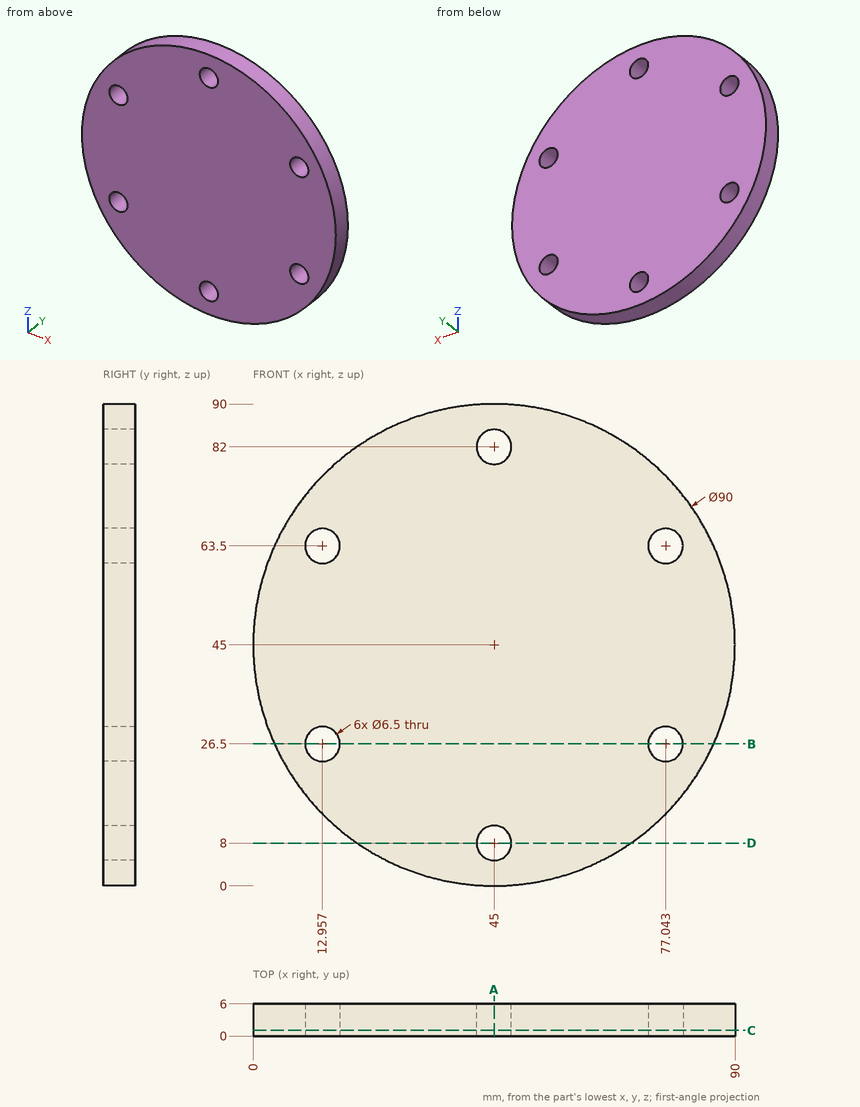
Here's the drawing with two shaded views (mm, measured from the low corner). I have some questions. Give positions to 0.01 mm unless a question says otherwise; leave off trailing zeros. Loops run counter-clockwise (first coordinate to the right, second up) from the corner with the lowest first, then second, coordinate; pieces in that order, holes last. Notation, with made-up numbers: (-5.75, 11.5) -> (13.25, 11.5) arc R15 cw to (13.25, 39.5) -> close; hole circle Ø9 at (-17.5, -36.75). An arc over 180 degrees is marked (long way). One line per item, written item: value.
Q1. Suppose I cut it at A-A on x = 45. Please give me the cut outline in (y, z).
Answers follow:
outline: (0, 0) -> (6, 0) -> (6, 4.75) -> (0, 4.75) -> close; (0, 11.25) -> (6, 11.25) -> (6, 78.75) -> (0, 78.75) -> close; (0, 85.25) -> (6, 85.25) -> (6, 90) -> (0, 90) -> close
Q2. If I drill on line 1 along Z through (x, y) = (45, 0.5); line 2 along X through (y, z) = (1.35, 29); line 3 along Z through (x, y) = (48, 3.2), over which ranges is the centre line in solid material (lowest first)?
Answers follow:
line 1: 0 to 4.75, 11.25 to 78.75, 85.25 to 90
line 2: 2.94 to 10.88, 15.03 to 74.97, 79.12 to 87.06
line 3: 0.1 to 6.75, 9.25 to 80.75, 83.25 to 89.9
Q3. Suppose I cut it at C-C on y = 1.05. Please give me the cut outline in (x, z).
Answers follow:
outline: circle Ø90 at (45, 45); hole circle Ø6.5 at (12.96, 26.5); hole circle Ø6.5 at (12.96, 63.5); hole circle Ø6.5 at (45, 8); hole circle Ø6.5 at (45, 82); hole circle Ø6.5 at (77.04, 26.5); hole circle Ø6.5 at (77.04, 63.5)
Q4. Suppose I cut it at B-B on z = 26.5. Please give me the cut outline in (x, y), then the cut area to 3 significant figures.
Answers follow:
outline: (3.98, 0) -> (9.71, 0) -> (9.71, 6) -> (3.98, 6) -> close; (16.21, 0) -> (73.79, 0) -> (73.79, 6) -> (16.21, 6) -> close; (80.29, 0) -> (86.02, 0) -> (86.02, 6) -> (80.29, 6) -> close
area: 414 mm^2
Q5. I'm going to push flat-ended pins straight in: pin 1 Ø2 at (x, y) = (58.5, 3.5) entering from -Z; pin 2 Ø3 at (y, z) = (3.5, 22.5) entering from -X; pin 3 Ø2 at (y, z) = (4, 24) entering from -X. Where does each tip first touch, or does it pass through?
Answers follow:
pin 1: z = 1.77
pin 2: x = 5.2
pin 3: x = 4.69
Q6. Suppose I cut it at D-D on z = 8. Please give me the cut outline in (x, y).
Answers follow:
outline: (19.39, 0) -> (41.75, 0) -> (41.75, 6) -> (19.39, 6) -> close; (48.25, 0) -> (70.61, 0) -> (70.61, 6) -> (48.25, 6) -> close
